Geometry check sheet. Reference: drawing and pictorial views, mm from the part's lowest x, y, z. Round coordinates to 2 decimals unless told otherwise and drop trailing zeros. Write each loop counter-clockwise with the first axis right and the second up, starting at its lowest first coordinate (ties: lowest second). Pieces come first, ordered by that corner, then holes. Notation, with made-up numbers: M 63,0 L 96,0 A13 cw 96,19 Z; hole C 51,18 d10. An arc over 180 degrees is marked long. One line per question, with ' | ' between items.
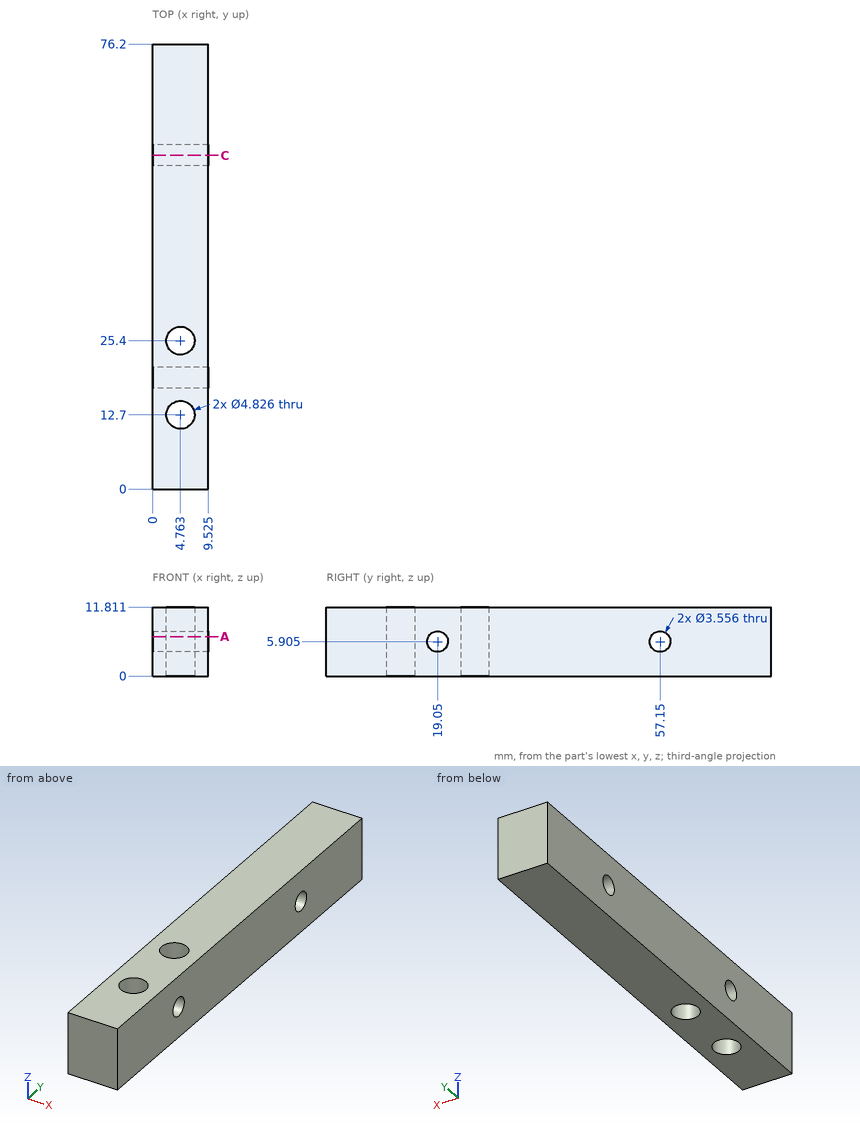
1. Section check C-C, the plane y = 57.15. Record the cut outline in (x, z) (1 decimal).
Results:
outline: M 0,0 L 9.5,0 L 9.5,4.1 L 0,4.1 Z; M 0,7.7 L 9.5,7.7 L 9.5,11.8 L 0,11.8 Z
2. Thickness scan on line 1 (Y direction, x = 5, z = 11); line 2 (Y direction, x = 5.5, z = 3); line 3 (Y direction, x = 4.25, z = 6) (1 decimal). Record the ranges inside material, lowest first.
Results:
line 1: y = 0 to 10.3, 15.1 to 23, 27.8 to 76.2 | line 2: y = 0 to 10.4, 15 to 23.1, 27.7 to 76.2 | line 3: y = 0 to 10.3, 15.1 to 17.3, 20.8 to 23, 27.8 to 55.4, 58.9 to 76.2
3. Section check A-A, the plane z = 6.75. Count the separate pieces of the cut face and the enclosed holes in it.
Results:
separate pieces: 3 | enclosed holes: 2
